from build123d import *
from OCP.BRepFilletAPI import BRepFilletAPI_MakeChamfer

# Parameters (mm, degrees)
EXTRUDE_1_DEPTH     = 150
SKETCH_2_R          = 5
CUT_EXTRUDE_2_DEPTH = 152.079449297
CHAMFER_1_SIZE      = 80
CHAMFER_1_SIZE2     = 2.094873726


with BuildPart() as part:
    # 草图1 → 拉伸1 (new body)
    with BuildSketch(Plane.XY):
        with BuildLine():
            Line((0, 10), (10, 10))
            ThreePointArc((10, 10), (15, 5), (10, 0))
            Line((10, 0), (0, 0))
            Line((0, 0), (0, 10))
        make_face()
    extrude(amount=EXTRUDE_1_DEPTH)

    # 草图2 → 拉伸2 (cut, through all)
    with BuildSketch(Plane(origin=(0, 10, 0), x_dir=(1, 0, 0), z_dir=(0, 1, 0))):
        with Locations(Location((7.5, -7.5, 0), (0, 0, 300))):
            Circle(SKETCH_2_R)
    extrude(amount=-CUT_EXTRUDE_2_DEPTH, mode=Mode.SUBTRACT)

    # 倒角1: one chamfer whose edges measure the first distance from different faces: ONE call of the kernel's chamfer builder (chamfer() names one face for all edges)
    chamfer_1_edges_1 = [part.edges().sort_by_distance(p)[0] for p in [
        (15, 5, 150),
    ]]
    chamfer_1_side_1 = [part.faces().sort_by_distance(p)[0] for p in [
        (15, 5, 75),
    ]]
    chamfer_1_edges_2 = [part.edges().sort_by_distance(p)[0] for p in [
        (5, 10, 150),
    ]]
    chamfer_1_side_2 = [part.faces().sort_by_distance(p)[0] for p in [
        (4.927731535, 10, 77.968371884),
    ]]
    chamfer_1_edges_3 = [part.edges().sort_by_distance(p)[0] for p in [
        (5, 0, 150),
    ]]
    chamfer_1_side_3 = [part.faces().sort_by_distance(p)[0] for p in [
        (4.927731535, 0, 77.968371884),
    ]]
    chamfer_1 = BRepFilletAPI_MakeChamfer(part.part.solid().wrapped)
    for e in chamfer_1_edges_1:
        chamfer_1.Add(CHAMFER_1_SIZE, CHAMFER_1_SIZE2, e.wrapped, chamfer_1_side_1[0].wrapped)  # the first distance lies on this face
    for e in chamfer_1_edges_2:
        chamfer_1.Add(CHAMFER_1_SIZE, CHAMFER_1_SIZE2, e.wrapped, chamfer_1_side_2[0].wrapped)  # the first distance lies on this face
    for e in chamfer_1_edges_3:
        chamfer_1.Add(CHAMFER_1_SIZE, CHAMFER_1_SIZE2, e.wrapped, chamfer_1_side_3[0].wrapped)  # the first distance lies on this face
    add(Compound.cast(chamfer_1.Shape()), mode=Mode.REPLACE)


solid = part.part
Verification items for the finished model (mm, model axes). A direction names the side the tool comes from. Give positions to 0.01 mm unless a question says otherwise; leave off trailing zeros. Loops run counter-clockwise (first coordinate to the right, second up) from the corner with the lowest first, then second, coordinate; pieces in that order, holes last. Notation, with made-up numbers: (-34, 81) - (-11, 81) arc R23 ccw to (-11, 97) - close; hole circle Ø6 at (-32.5, 39.25). An arc over 180 degrees is marked (long way). Write item = value, one per line. Start each with the question number.
Q1. Cross-section at B-B, the plane z = 7.5. Enter the section's corners in (x, y), and give its area (3 significant figures).
Q2. Depth check by flat-ended pin: P1, Ø1.5, axis at x = 6.5, z = 90, coming from the -Y side; P2, Ø2, axis at y = 4.5, z = 124.5, coming from the +X side; P3, Ø1, axis at x = 2.5, z = 102, coming from the +Y side. Enter the tip coordinate at first touch or a pass-through.
Q3. Thickness scan on line 1 (Z direction, x = 7.5, y = 3.5); line 2 (X direction, y = 6.25, z = 7.5); line 3 (Z direction, x = 10.5, y = 3.75). Record the ranges inside material, lowest first.
Q4. Cross-section at C-C, the plane y = 5. Enter the section's corners in (x, z).
Q5. Cross-section at A-A, the plane x = 7.5. Enter the section's corners in (y, z), and give its area (3 significant figures).
Q6. Tool access check on faces 4 (the face through (5, 0, 35)), 5 (the face through (13.937, 5.087, 110.56)). Record the directions out of +Z, -Z, +X, -X, +Y, -Y that give a thin tool (end or side, any length) a straight path to the whole face; none if there is none.
Q7. Cross-section at D-D, the plane z = 133. Enter the section's corners in (x, y).
Q8. Mould release check, pull along X, two halves, no side actions. Record for faces 1 (the face through (8, 5, 0)), 2 (the face through (2.881, 5.07, 5.585)), 3 (the face through (15, 5, 35)): released by +X, released by -X, zero draft, split by the parting line, or undercut.
Answer key:
q1.outline = (0, 0) - (2.5, 0) - (2.5, 10) - (0, 10) - close; (12.5, 0.67) arc R5 ccw to (12.5, 9.33) - close
q1.area = 40.4 mm^2
q2.P1 = 0.5
q2.P2 = 13.6
q2.P3 = 9.18
q3.line_1 = 0 to 2.5, 12.5 to 150
q3.line_2 = 0 to 2.5, 12.5 to 14.84
q3.line_3 = 0 to 3.5, 11.5 to 150
q4.outline = (0, 0) - (15, 0) - (15, 70) - (12.91, 150) - (0, 150) - close; hole circle Ø10 at (7.5, 7.5)
q5.outline = (0, 0) - (10, 0) - (10, 2.5) - (0, 2.5) - close; (0, 12.5) - (10, 12.5) - (10, 70) - (7.91, 150) - (2.09, 150) - (0, 70) - close
q5.area = 1,230 mm^2
q6.face_4 = +Z, -Z, +X, -X, -Y
q6.face_5 = +Z, +X
q7.outline = (0, 1.65) - (10, 1.65) arc R3.35 ccw to (10, 8.35) - (0, 8.35) - close
q8.face_1 = zero draft
q8.face_2 = undercut
q8.face_3 = released by +X
